```python
from build123d import *

# Parameters (mm, degrees)
EXTRUSION1_DEPTH = 70
EXTRUSION2_REACH = 3
ESQUISSE2_R      = 2
EXTRUSION3_REACH = 13.207
ESQUISSE3_R      = 2


with BuildPart() as part:
    # Esquisse1 → Extrusion1 (new body)
    with BuildSketch(Plane(origin=(0, 0, 0), x_dir=(1, 0, 0), z_dir=(0, 1, 0))):
        Polygon((0, 0), (0, 20.414213562), (1, 20.414213562), (1, 0.414213562), (15.142135624, -13.727922061), (14.435028843, -14.435028843), align=None)
    extrude(amount=EXTRUSION1_DEPTH)

    # Esquisse2 → Extrusion2 (cut, up to next)
    with BuildSketch(Plane(origin=(1, 0, 0), x_dir=(0, 0, -1), z_dir=(1, 0, 0)), mode=Mode.PRIVATE) as extrusion2_sk1:
        with Locations((10.414213562, 16.5)):
            Circle(ESQUISSE2_R)
    extrusion2_tool1 = extrude(extrusion2_sk1.sketch, amount=-EXTRUSION2_REACH, mode=Mode.PRIVATE) & part.part
    add(extrusion2_tool1.solids().sort_by_distance((1, 16.5, -10.414214))[0], mode=Mode.SUBTRACT)
    # Esquisse2 → Extrusion2 (cut, up to next)
    with BuildSketch(Plane(origin=(1, 0, 0), x_dir=(0, 0, -1), z_dir=(1, 0, 0)), mode=Mode.PRIVATE) as extrusion2_sk2:
        with Locations((10.414213562, 6.5)):
            Circle(ESQUISSE2_R)
    extrusion2_tool2 = extrude(extrusion2_sk2.sketch, amount=-EXTRUSION2_REACH, mode=Mode.PRIVATE) & part.part
    add(extrusion2_tool2.solids().sort_by_distance((1, 6.5, -10.414214))[0], mode=Mode.SUBTRACT)
    # Esquisse2 → Extrusion2 (cut, up to next)
    with BuildSketch(Plane(origin=(1, 0, 0), x_dir=(0, 0, -1), z_dir=(1, 0, 0)), mode=Mode.PRIVATE) as extrusion2_sk3:
        with Locations((10.414213562, 53.5)):
            Circle(ESQUISSE2_R)
    extrusion2_tool3 = extrude(extrusion2_sk3.sketch, amount=-EXTRUSION2_REACH, mode=Mode.PRIVATE) & part.part
    add(extrusion2_tool3.solids().sort_by_distance((1, 53.5, -10.414214))[0], mode=Mode.SUBTRACT)
    # Esquisse2 → Extrusion2 (cut, up to next)
    with BuildSketch(Plane(origin=(1, 0, 0), x_dir=(0, 0, -1), z_dir=(1, 0, 0)), mode=Mode.PRIVATE) as extrusion2_sk4:
        with Locations((10.414213562, 63.5)):
            Circle(ESQUISSE2_R)
    extrusion2_tool4 = extrude(extrusion2_sk4.sketch, amount=-EXTRUSION2_REACH, mode=Mode.PRIVATE) & part.part
    add(extrusion2_tool4.solids().sort_by_distance((1, 63.5, -10.414214))[0], mode=Mode.SUBTRACT)

    # Esquisse3 → Extrusion3 (cut, up to next)
    with BuildSketch(Plane(origin=(0.707106781, 0, -0.707106781), x_dir=(-0.707106781, 0, -0.707106781), z_dir=(0.707106781, 0, -0.707106781)), mode=Mode.PRIVATE) as extrusion3_sk1:
        with Locations((-10.414213562, 53.5)):
            Circle(ESQUISSE3_R)
    extrusion3_tool1 = extrude(extrusion3_sk1.sketch, amount=-EXTRUSION3_REACH, mode=Mode.PRIVATE) & part.part
    add(extrusion3_tool1.solids().sort_by_distance((8.071068, 53.5, 6.656854))[0], mode=Mode.SUBTRACT)
    # Esquisse3 → Extrusion3 (cut, up to next)
    with BuildSketch(Plane(origin=(0.707106781, 0, -0.707106781), x_dir=(-0.707106781, 0, -0.707106781), z_dir=(0.707106781, 0, -0.707106781)), mode=Mode.PRIVATE) as extrusion3_sk2:
        with Locations((-10.414213562, 63.5)):
            Circle(ESQUISSE3_R)
    extrusion3_tool2 = extrude(extrusion3_sk2.sketch, amount=-EXTRUSION3_REACH, mode=Mode.PRIVATE) & part.part
    add(extrusion3_tool2.solids().sort_by_distance((8.071068, 63.5, 6.656854))[0], mode=Mode.SUBTRACT)
    # Esquisse3 → Extrusion3 (cut, up to next)
    with BuildSketch(Plane(origin=(0.707106781, 0, -0.707106781), x_dir=(-0.707106781, 0, -0.707106781), z_dir=(0.707106781, 0, -0.707106781)), mode=Mode.PRIVATE) as extrusion3_sk3:
        with Locations((-10.414213562, 6.5)):
            Circle(ESQUISSE3_R)
    extrusion3_tool3 = extrude(extrusion3_sk3.sketch, amount=-EXTRUSION3_REACH, mode=Mode.PRIVATE) & part.part
    add(extrusion3_tool3.solids().sort_by_distance((8.071068, 6.5, 6.656854))[0], mode=Mode.SUBTRACT)
    # Esquisse3 → Extrusion3 (cut, up to next)
    with BuildSketch(Plane(origin=(0.707106781, 0, -0.707106781), x_dir=(-0.707106781, 0, -0.707106781), z_dir=(0.707106781, 0, -0.707106781)), mode=Mode.PRIVATE) as extrusion3_sk4:
        with Locations((-10.414213562, 16.5)):
            Circle(ESQUISSE3_R)
    extrusion3_tool4 = extrude(extrusion3_sk4.sketch, amount=-EXTRUSION3_REACH, mode=Mode.PRIVATE) & part.part
    add(extrusion3_tool4.solids().sort_by_distance((8.071068, 16.5, 6.656854))[0], mode=Mode.SUBTRACT)


solid = part.part
```
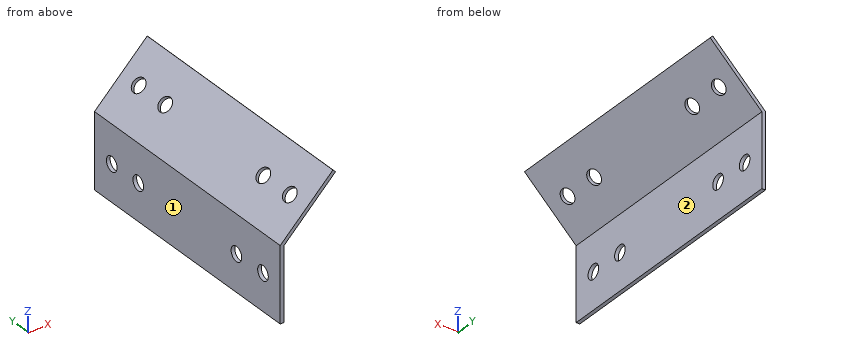
Geometry check sheet. Reference: the model listing, model coordinates, mm. Face numbers are marked on the shaded views. A direction names the side the tool comes from. Give positions to 0.01 mm unless a question says otherwise; leave off trailing zeros. Order: outer loops, then holes, each group sorted by start corner. A loop starts at its lowest first (then second) coordinate and runs counter-clockwise, first axis right, second up.
1. Section check A-A, the plane y = 53.5. Enter the section's corners in (x, z), and give its area (3 significant figures).
2. Thickness scan on L1, parallel to X at y = 43.5, z = -12; L2, parallel to X at y = 55, z = 4.5; L3, parallel to Z at x = 0.75, y = 40.5. Record the ranges inside material, lowest first.
3. Access from +Z, -Z, +X, -X, +Y, -Y to the whole of each face (thin tool, end or side, straight path). Record for the marked faces 1 and 2.
4. Gauge pin test, flat ends, axial feed: pin 1 Ø3.5 at (y, z) = (63.5, -10.41) entering from +X; pin 2 Ø1.5 at (y, z) = (38.5, -11.5) entering from +X; pin 3 Ø1.5 at (y, z) = (50, 8.5) entering from -X; pin 4 Ø5 at (y, z) = (47, -2.5) entering from +X. Record the tip position at first contact, or that the pin passes through.
5. Section check B-B, the plane y = 21. Enter the section's corners in (x, z), and give its area (3 significant figures).
6. Section check C-C, the plane z = 7. Give the number of separate pieces and of enclosed holes in the cut face, and give its area (3 significant figures).
Values follow:
1. outline: (0, -20.41) - (1, -20.41) - (1, -12.41) - (0, -12.41) - close; (0, -8.41) - (1, -8.41) - (1, -0.41) - (6.66, 5.24) - (5.95, 5.95) - (0, 0) - close; (8.78, 8.78) - (9.49, 8.07) - (15.14, 13.73) - (14.44, 14.44) - close
1. area: 32.4 mm2
2. L1: x = 0 to 1
2. L2: x = 4.5 to 5.91
2. L3: z = -20.41 to 0.75
3. face 1: +Z, -Z, -X, +Y, -Y
3. face 2: -Z, +X, +Y, -Y
4. pin 1: passes through
4. pin 2: stops at x = 1
4. pin 3: stops at x = 7.75
4. pin 4: stops at x = 1.41
5. outline: (0, -20.41) - (1, -20.41) - (1, -0.41) - (15.14, 13.73) - (14.44, 14.44) - (0, 0) - close
5. area: 40.4 mm2
6. separate pieces: 5
6. enclosed holes: 0
6. area: 76.6 mm2
